```python
from build123d import *

# Parameters (mm, degrees)
SKETCH_1_W          = 36
SKETCH_1_H          = 21
SKETCH_1_R          = 1.25
SKETCH_1_R_2        = 1.3
SKETCH_1_R_3        = 1.35
EXTRUDE_1_DEPTH     = 90
SKETCH_1_5_R        = 1.3
SKETCH_1_5_R_2      = 1.35
SKETCH_1_5_R_3      = 1.25
CUT_EXTRUDE_1_DEPTH = 4
CUT_EXTRUDE_START   = 90
SKETCH_1_6_R        = 1.35
SKETCH_1_6_R_2      = 1.3
SKETCH_1_6_R_3      = 1.25
CUT_EXTRUDE_2_DEPTH = 4
CUT_EXTRUDE_3_REACH = 96.154
FILLET_1_R          = 1.5


with BuildPart() as part:
    # 스케치1 → 보스-돌출1 (new body)
    with BuildSketch(Plane.XY):
        Rectangle(SKETCH_1_W, SKETCH_1_H)
        with Locations((-3.5, -8)):
            Circle(SKETCH_1_R, mode=Mode.SUBTRACT)
        with Locations((3.5, -8)):
            Circle(SKETCH_1_R, mode=Mode.SUBTRACT)
        with Locations((-12, 6)):
            Circle(SKETCH_1_R_2, mode=Mode.SUBTRACT)
        with Locations((12, 6)):
            Circle(SKETCH_1_R_2, mode=Mode.SUBTRACT)
        with Locations((12, -6)):
            Circle(SKETCH_1_R_2, mode=Mode.SUBTRACT)
        with Locations((-12, -6)):
            Circle(SKETCH_1_R_2, mode=Mode.SUBTRACT)
        with Locations((3.5, 8)):
            Circle(SKETCH_1_R_3, mode=Mode.SUBTRACT)
        with Locations((-3.5, 8)):
            Circle(SKETCH_1_R_3, mode=Mode.SUBTRACT)
        with Locations((12, -6)):
            Circle(SKETCH_1_R_2)
        with Locations((3.5, -8)):
            Circle(SKETCH_1_R)
        with Locations((-3.5, -8)):
            Circle(SKETCH_1_R)
        with Locations((-12, -6)):
            Circle(SKETCH_1_R_2)
        with Locations((-12, 6)):
            Circle(SKETCH_1_R_2)
        with Locations((-3.5, 8)):
            Circle(SKETCH_1_R_3)
        with Locations((3.5, 8)):
            Circle(SKETCH_1_R_3)
        with Locations((12, 6)):
            Circle(SKETCH_1_R_2)
    extrude(amount=EXTRUDE_1_DEPTH)

    # 스케치1<5> → 컷-돌출1 (cut)
    with BuildSketch(Plane.XY):
        with Locations((12, 6)):
            Circle(SKETCH_1_5_R)
        with Locations((3.5, 8)):
            Circle(SKETCH_1_5_R_2)
        with Locations((-3.5, 8)):
            Circle(SKETCH_1_5_R_2)
        with Locations((-12, 6)):
            Circle(SKETCH_1_5_R)
        with Locations((-12, -6)):
            Circle(SKETCH_1_5_R)
        with Locations(Location((-3.5, -8, 0), (0, 0, 180))):
            Circle(SKETCH_1_5_R_3)
        with Locations((3.5, -8)):
            Circle(SKETCH_1_5_R_3)
        with Locations((12, -6)):
            Circle(SKETCH_1_5_R)
    extrude(amount=CUT_EXTRUDE_1_DEPTH, mode=Mode.SUBTRACT)

    # 스케치1<6> → 컷-돌출2 (cut)
    with BuildSketch(Plane.XY.offset(CUT_EXTRUDE_START)):
        with Locations((3.5, 8)):
            Circle(SKETCH_1_6_R)
        with Locations((12, 6)):
            Circle(SKETCH_1_6_R_2)
        with Locations((-3.5, 8)):
            Circle(SKETCH_1_6_R)
        with Locations((-12, 6)):
            Circle(SKETCH_1_6_R_2)
        with Locations((-12, -6)):
            Circle(SKETCH_1_6_R_2)
        with Locations(Location((-3.5, -8, 0), (0, 0, 180))):
            Circle(SKETCH_1_6_R_3)
        with Locations((3.5, -8)):
            Circle(SKETCH_1_6_R_3)
        with Locations((12, -6)):
            Circle(SKETCH_1_6_R_2)
    extrude(amount=-CUT_EXTRUDE_2_DEPTH, mode=Mode.SUBTRACT)

    # 스케치2 → 컷-돌출3 (cut, up to next)
    with BuildSketch(Plane(origin=(0, 10.5, 0), x_dir=(1, 0, 0), z_dir=(0, 1, 0)), mode=Mode.PRIVATE) as cut_extrude_3_sk1:
        with BuildLine():
            Line((7.5, -15), (7.5, -75))
            ThreePointArc((7.5, -75), (0, -82.5), (-7.5, -75))
            Line((-7.5, -75), (-7.5, -15))
            ThreePointArc((-7.5, -15), (0, -7.5), (7.5, -15))
        make_face()
    cut_extrude_3_tool1 = extrude(cut_extrude_3_sk1.sketch, amount=-CUT_EXTRUDE_3_REACH, mode=Mode.PRIVATE) & part.part
    add(cut_extrude_3_tool1.solids().sort_by_distance((0, 10.5, 45))[0], mode=Mode.SUBTRACT)

    # 필렛1
    fillet_1_edges = [part.edges().sort_by_distance(p)[0] for p in [
        (0, -10.5, 7.5),
        (7.5, -10.5, 45),
        (0, -10.5, 82.5),
        (-7.5, -10.5, 45),
        (0, 10.5, 7.5),
        (-7.5, 10.5, 45),
        (0, 10.5, 82.5),
        (7.5, 10.5, 45),
        (-18, 10.5, 45),
        (18, 10.5, 45),
        (18, -10.5, 45),
        (-18, -10.5, 45),
    ]]
    fillet(fillet_1_edges, radius=FILLET_1_R)


solid = part.part
```
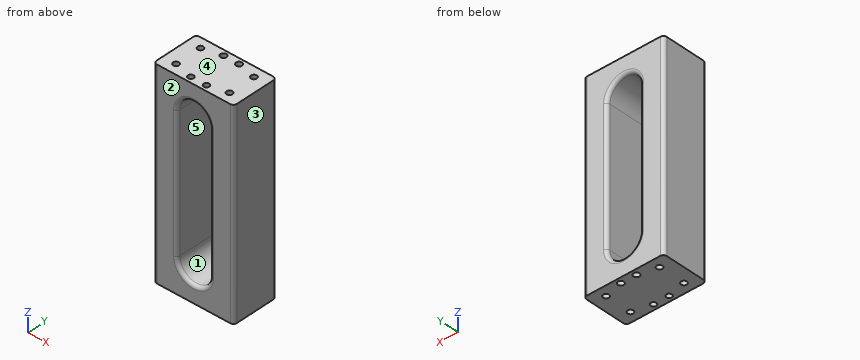
Source: CAD feature listing. Evaluate the final solid. Frame: model axes, mm. Face numbers are marked on the shaded views. A direction names the side the tool comes from. Coordinates: 2 decimals unless noted, no trailing zeros. Write each loop counter-clockwise with the first axis right and the second up, starting at its lowest first coordinate (ties: lowest second). Pieces come first, ordered by that corner, then holes. Notation, with made-up numbers: (-4, 45.5) - (18, 45.5) arc R4 ccw to (18, 50.5) - close; hole circle Ø10 at (62, -2). An arc over 180 degrees is marked (long way). Answer as a JSON object with one key per item and string values.
Q1. Section query D-D, the plane x = 12. Output: boundary loops of the cut face in (y, z).
Ans:
{"outline": "(-10.5, 0) - (-7.3, 0) - (-7.3, 4) - (-4.7, 4) - (-4.7, 0) - (4.7, 0) - (4.7, 4) - (7.3, 4) - (7.3, 0) - (10.5, 0) - (10.5, 90) - (7.3, 90) - (7.3, 86) - (4.7, 86) - (4.7, 90) - (-4.7, 90) - (-4.7, 86) - (-7.3, 86) - (-7.3, 90) - (-10.5, 90) - close"}
Q2. Section query B-B, the plane y = 0. Output: boundary loops of the cut face in (x, z).
Ans:
{"outline": "(-18, 0) - (18, 0) - (18, 90) - (-18, 90) - close; hole (-7.5, 15) arc R7.5 ccw to (7.5, 15) - (7.5, 75) arc R7.5 ccw to (-7.5, 75) - close"}
Q3. Draft query along X for the marked faces 1, 2 and 3. Return one class per face: released by +X, released by -X, zero draft, split by the parting line, or undercut.
Ans:
{"face 1": "undercut", "face 2": "zero draft", "face 3": "released by +X"}
Q4. Set-up query: the marked faces 4 and 5. Return all of +Z, -Z, +X, -X, +Y, -Y with unobstructed straight access to the full face (end or side cutting, diameter ignored); none if empty.
Ans:
{"face 4": "+Z, +X, -X, +Y, -Y", "face 5": "+Y, -Y"}
Q5. Section query A-A, the plane x = 0. Output: boundary loops of the cut face in (y, z).
Ans:
{"outline": "(-10.5, 0) - (10.5, 0) - (10.5, 6) arc R1.5 ccw to (9, 7.5) - (-9, 7.5) arc R1.5 ccw to (-10.5, 6) - close; (-10.5, 84) arc R1.5 ccw to (-9, 82.5) - (9, 82.5) arc R1.5 ccw to (10.5, 84) - (10.5, 90) - (-10.5, 90) - close"}
Q6. Section query C-C, the plane z = 37.5. Output: boundary loops of the cut face in (x, y).
Ans:
{"outline": "(-18, -9) arc R1.5 ccw to (-16.5, -10.5) - (-9, -10.5) arc R1.5 ccw to (-7.5, -9) - (-7.5, 9) arc R1.5 ccw to (-9, 10.5) - (-16.5, 10.5) arc R1.5 ccw to (-18, 9) - close; (7.5, -9) arc R1.5 ccw to (9, -10.5) - (16.5, -10.5) arc R1.5 ccw to (18, -9) - (18, 9) arc R1.5 ccw to (16.5, 10.5) - (9, 10.5) arc R1.5 ccw to (7.5, 9) - close"}
Q7. First-contact query: pin 1 Ø0.8 at (x, y) = (-4, -7.5) entering from -Z; pin 2 Ø12 at (x, y) = (12.5, -7) entering from -Z; pin 3 Ø1.2 at (x, y) = (-4, -8) entering from +Z. Flat tips, straight axial feed; report the tip coordinate or a pass-through.
Ans:
{"pin 1": "stops at z = 4", "pin 2": "stops at z = 0", "pin 3": "stops at z = 86"}
Q8. Material intervals for line 1 (Y direction, x = -3.5, z = 1.5); line 2 (Y direction, x = -12, z = 87.2); line 3 (X direction, y = 6.5, z = 68.5), sorted ascending. Write a range as [from, to].
Ans:
{"line 1": "y = [-10.5, -9.25], [-6.75, 6.65], [9.35, 10.5]", "line 2": "y = [-10.5, -7.3], [-4.7, 4.7], [7.3, 10.5]", "line 3": "x = [-18, -7.5], [7.5, 18]"}
